```python
from build123d import *

# Parameters (mm, degrees)
ESBO_O1_R                = 4
ESBO_O1_R_2              = 1.5
ESBO_O1_R_3              = 4.5
ESBO_O1_W                = 6.25
ESBO_O1_H                = 8.25
RESSALTO_EXTRUS_O1_DEPTH = 6


with BuildPart() as part:
    # Esboço1 → Ressalto-extrusão1 (new body)
    with BuildSketch(Plane.XY):
        with BuildLine():
            Line((50, -7), (50, 15))
            Line((50, 15), (-106, 15))
            Line((-106, 15), (-106, 25))
            Line((-106, 25), (-130, 25))
            Line((-130, 25), (-130, -7))
            ThreePointArc((-130, -7), (-118, -19), (-106, -7))
            Line((-106, -7), (-35, -7))
            ThreePointArc((-35, -7), (-35.454682684, -15.675862451), (-36.813749139, -24.256670338))
            Line((-36.813749139, -24.256670338), (-30.944863535, -25.504140483))
            ThreePointArc((-30.944863535, -25.504140483), (-30.499970699, -23.270982524), (-30.112353587, -21.027173913))
            ThreePointArc((-30.112353587, -21.027173913), (-26.677022565, -18.537495065), (-24.187343716, -21.972826087))
            ThreePointArc((-24.187343716, -21.972826087), (-24.601092319, -24.367902694), (-25.07597793, -26.751610628))
            Line((-25.07597793, -26.751610628), (-19.207092326, -27.999080773))
            ThreePointArc((-19.207092326, -27.999080773), (-17.553288568, -17.55737479), (-17, -7))
            Line((-17, -7), (50, -7))
        make_face()
        with Locations((-118, -7)):
            Circle(ESBO_O1_R, mode=Mode.SUBTRACT)
        with Locations((-70, 5)):
            Circle(ESBO_O1_R_2, mode=Mode.SUBTRACT)
        with Locations((40, 5)):
            Circle(ESBO_O1_R_2, mode=Mode.SUBTRACT)
        with Locations((-87.5, 9)):
            Circle(ESBO_O1_R_3, mode=Mode.SUBTRACT)
        with Locations((-118, 15.875)):
            Rectangle(ESBO_O1_W, ESBO_O1_H, mode=Mode.SUBTRACT)
    extrude(amount=RESSALTO_EXTRUS_O1_DEPTH)


solid = part.part
```
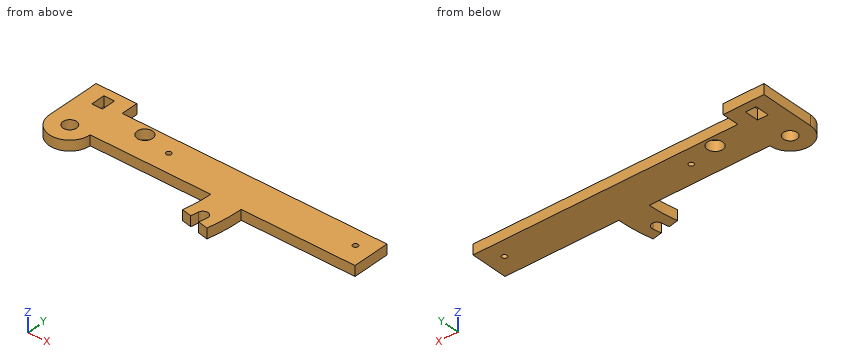
Here's how the part is built. I have some questions about the finished solid (model axes, mm). Give positions to 0.01 mm unless a question says otherwise; leave off trailing zeros. Order: outer loops, then holes, each group sorted by start corner. A loop starts at its lowest first (then second) coordinate and runs counter-clockwise, first axis right, second up. Notation, with made-up numbers: M 30,31.25 L 44,31.25 A20 ccw 44,56.25 Z; hole C 41.25,-16 d10. An arc over 180 degrees is marked long. Use a Markdown table: item, result. Add a question column.
1. Suppose I cut it at A-A (y = 9). List the corners of the cut face in (x, z) for me.
2. Suppose I cut it at C-C (x = 24). List the corners of the cut face in (y, z) for me.
3. I need wall thicknesses on probe 1 along Y at (x, z) = (-118, 3.65); probe 2 along Y at (x, z) = (-70, 2.1); probe 3 along X at (y, z) = (-6.5, 4.25). Which ranges of each line are inside material? Lowest first, please. Write a range as from..to.
4. For pin 1 Ø1.5 at (x, z) = (-6, 3.5) entering from -Y; pin 2 Ø2.5 at (x, y) = (-70, 5) entering from -Z; pin 3 Ø3 at (x, z) = (21, 0.5) entering from +Y, each with a flat end and sliding along its axis, tell me the tip position at first contact or that it passes through.
5. Suppose I cut it at B-B (z = 4.3). List the corners of the cut face in (x, y) for me (3 decimals).
Results list:
| question | item | result |
|---|---|---|
| 1 | outline | M -130,0 L -92,0 L -92,6 L -130,6 Z; M -83,0 L 50,0 L 50,6 L -83,6 Z |
| 2 | outline | M -7,0 L 15,0 L 15,6 L -7,6 Z |
| 3 | probe 1 | y = -19..-11, -3..11.75, 20..25 |
| 3 | probe 2 | y = -7..3.5, 6.5..15 |
| 3 | probe 3 | x = -130..-121.97, -114.03..50 |
| 4 | pin 1 | stops at y = -7 |
| 4 | pin 2 | passes through |
| 4 | pin 3 | stops at y = 15 |
| 5 | outline | M -130,-7 A12 ccw -106,-7 L -35,-7 A83 cw -36.814,-24.257 L -30.945,-25.504 A89 ccw -30.112,-21.027 A3 cw -24.187,-21.973 A95 cw -25.076,-26.752 L -19.207,-27.999 A101 ccw -17,-7 L 50,-7 L 50,15 L -106,15 L -106,25 L -130,25 Z; hole C -118,-7 d8; hole M -121.125,11.75 L -114.875,11.75 L -114.875,20 L -121.125,20 Z; hole C -87.5,9 d9; hole C -70,5 d3; hole C 40,5 d3 |
